Geometry check sheet. Reference: the model listing, model coordinates, mm. Face numbers are marked on the shaded views. A direction names the side the tool comes from. Round coordinates to 2 decimals unless told otherwise and drop trailing zeros. Write each loop counter-clockwise with the first axis right and the second up, starting at its lowest first coordinate (ties: lowest second). Pieces come first, ordered by that corner, then holes. Notation, with made-up numbers: M 79,64 L 135,64 A22 cw 135,87 Z; hole C 68,43.5 d8. An arc over 180 degrees is marked long. Put each result on its own line as item: value. Start each with the question number.
(1) Section check A-A on z = 64. Record the cut outline in (x, y).
(2) Mould release check, pull along Y, two halves, no side actions. Record for the marked faces 3, 4 and 5: pulls with the +Y half, pulls with the -Y half, needs draft (parallel to the pull), parting line crosses it, or undercut.
(3) Section check C-C on x = 37.5. Record the cut outline in (y, z).
(4) Gauge pin test, flat ends, axial feed: pin 1 (5 mm diameter, centred on x = 45, z = 17, fed in from -Y); pin 2 (4 mm diameter, centred on x = 4, z = 22.5, fed in from +Y); pin 3 (4 mm diameter, centred on x = 4, z = 27, fed in from -Y); pin 4 (3 mm diameter, centred on y = 33.5, z = 80.5, fed in from +X). Record the tip position at first contact, or that the pin passes through.
(5) Tool access check on the marked faces 1 and 2. Record the directions out of +Z, -Z, +X, -X, +Y, -Y that give a thin tool (end or side, any length) a straight path to the whole face; none if there is none.
(6) Section check D-D on z = 7. Record the cut outline in (x, y), then the cut area to 3 significant figures.
(7) Section check B-B on y = 36. Record the cut outline in (x, z).
(8) Material ranges on probe 1 along X at (y, z) = (4, 72.5); probe 2 along Z at (x, y) = (14.5, 33.5); probe 3 along X at (y, z) = (51, 35), recorded low to high.
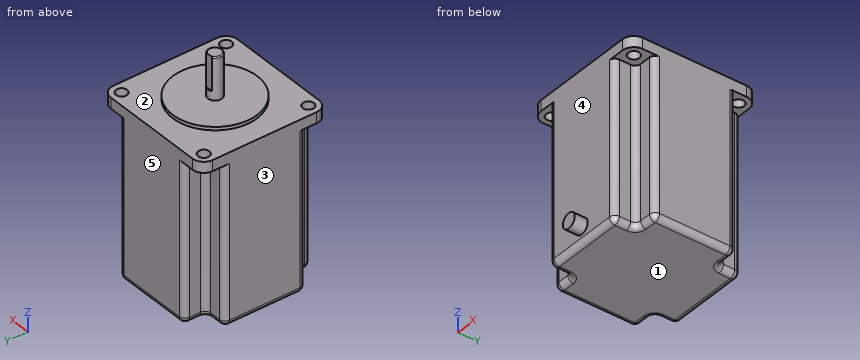
from build123d import *

# Parameters (mm, degrees)
SKETCH1_W           = 57.15
SKETCH1_H           = 57.15
BOSS_EXTRUDE1_DEPTH = 76.2
SKETCH2_R           = 19.05
BOSS_EXTRUDE2_DEPTH = 1.524
SKETCH3_R           = 3.175
BOSS_EXTRUDE3_DEPTH = 19.05
SKETCH18_W          = 20.32
SKETCH18_H          = 20.32
CUT_EXTRUDE13_DEPTH = 71.3232
SKETCH20_W          = 20.32
SKETCH20_H          = 20.32
CUT_EXTRUDE14_DEPTH = 71.3232
SKETCH21_W          = 20.32
SKETCH21_H          = 20.32
CUT_EXTRUDE15_DEPTH = 71.3232
SKETCH22_W          = 20.32
SKETCH22_H          = 20.32
CUT_EXTRUDE16_DEPTH = 71.3232
SKETCH11_R          = 2.54
CUT_EXTRUDE8_DEPTH  = 112.079633597
SKETCH12_R          = 2.54
CUT_EXTRUDE9_DEPTH  = 112.079633597
SKETCH14_R          = 2.54
CUT_EXTRUDE10_DEPTH = 112.079633597
SKETCH15_R          = 2.54
CUT_EXTRUDE11_DEPTH = 112.079633597
FILLET2_R           = 5.08
FILLET4_R           = 2.54
FILLET1_R           = 0.508
SKETCH10_W          = 7.148953117
SKETCH10_H          = 1.106198654
CUT_EXTRUDE7_DEPTH  = 14.986
SKETCH23_R          = 3.429
WIRE_2_DEPTH        = 5.842


with BuildPart() as part:
    # Sketch1 → Boss-Extrude1 (new body)
    with BuildSketch(Plane.XY):
        with Locations((28.575, 28.575)):
            Rectangle(SKETCH1_W, SKETCH1_H)
    extrude(amount=BOSS_EXTRUDE1_DEPTH)

    # Sketch2 → Boss-Extrude2 (add)
    with BuildSketch(Plane.XY.offset(76.2)):
        with Locations(Location((28.575, 28.575, 0), (0, 0, 180))):
            Circle(SKETCH2_R)
    extrude(amount=BOSS_EXTRUDE2_DEPTH)

    # Sketch3 → Boss-Extrude3 (add)
    with BuildSketch(Plane.XY.offset(77.724)):
        with Locations(Location((28.575, 28.575, 0), (0, 0, 180))):
            Circle(SKETCH3_R)
    extrude(amount=BOSS_EXTRUDE3_DEPTH)

    # Sketch18 → Cut-Extrude13 (cut)
    with BuildSketch(Plane(origin=(0, 0, 0), x_dir=(-1, 0, 0), z_dir=(0, 0, -1))):
        with Locations((0, 57.15)):
            Rectangle(SKETCH18_W, SKETCH18_H)
    extrude(amount=-CUT_EXTRUDE13_DEPTH, mode=Mode.SUBTRACT)

    # Sketch20 → Cut-Extrude14 (cut)
    with BuildSketch(Plane(origin=(0, 0, 0), x_dir=(-1, 0, 0), z_dir=(0, 0, -1))):
        Rectangle(SKETCH20_W, SKETCH20_H)
    extrude(amount=-CUT_EXTRUDE14_DEPTH, mode=Mode.SUBTRACT)

    # Sketch21 → Cut-Extrude15 (cut)
    with BuildSketch(Plane(origin=(0, 0, 0), x_dir=(-1, 0, 0), z_dir=(0, 0, -1))):
        with Locations((-57.15, 0)):
            Rectangle(SKETCH21_W, SKETCH21_H)
    extrude(amount=-CUT_EXTRUDE15_DEPTH, mode=Mode.SUBTRACT)

    # Sketch22 → Cut-Extrude16 (cut)
    with BuildSketch(Plane(origin=(0, 0, 0), x_dir=(-1, 0, 0), z_dir=(0, 0, -1))):
        with Locations((-57.15, 57.15)):
            Rectangle(SKETCH22_W, SKETCH22_H)
    extrude(amount=-CUT_EXTRUDE16_DEPTH, mode=Mode.SUBTRACT)

    # Sketch11 → Cut-Extrude8 (cut, through all)
    with BuildSketch(Plane.XY.offset(76.2)):
        with Locations((4.953, 52.233071325)):
            Circle(SKETCH11_R)
    extrude(amount=-CUT_EXTRUDE8_DEPTH, mode=Mode.SUBTRACT)

    # Sketch12 → Cut-Extrude9 (cut, through all)
    with BuildSketch(Plane.XY.offset(76.2)):
        with Locations((52.197, 52.233071325)):
            Circle(SKETCH12_R)
    extrude(amount=-CUT_EXTRUDE9_DEPTH, mode=Mode.SUBTRACT)

    # Sketch14 → Cut-Extrude10 (cut, through all)
    with BuildSketch(Plane.XY.offset(76.2)):
        with Locations((4.953, 4.989071325)):
            Circle(SKETCH14_R)
    extrude(amount=-CUT_EXTRUDE10_DEPTH, mode=Mode.SUBTRACT)

    # Sketch15 → Cut-Extrude11 (cut, through all)
    with BuildSketch(Plane.XY.offset(76.2)):
        with Locations((52.197, 4.989071325)):
            Circle(SKETCH15_R)
    extrude(amount=-CUT_EXTRUDE11_DEPTH, mode=Mode.SUBTRACT)

    # Fillet2
    fillet2_edges = [part.edges().sort_by_distance(p)[0] for p in [
        (0, 57.15, 73.7616),
        (57.15, 57.15, 73.7616),
        (57.15, 0, 73.7616),
        (0, 0, 73.7616),
    ]]
    fillet(fillet2_edges, radius=FILLET2_R)

    # Fillet4
    fillet4_edges = [part.edges().sort_by_distance(p)[0] for p in [
        (0, 28.575, 0),
        (10.16, 52.07, 0),
        (5.08, 46.99, 0),
        (0, 46.99, 35.6616),
        (10.16, 57.15, 35.6616),
        (10.16, 46.99, 35.6616),
        (28.575, 0, 0),
        (5.08, 10.16, 0),
        (10.16, 5.08, 0),
        (10.16, 0, 35.6616),
        (0, 10.16, 35.6616),
        (10.16, 10.16, 35.6616),
        (57.15, 28.575, 0),
        (46.99, 5.08, 0),
        (52.07, 10.16, 0),
        (57.15, 10.16, 35.6616),
        (46.99, 0, 35.6616),
        (46.99, 10.16, 35.6616),
        (28.575, 57.15, 0),
        (52.07, 46.99, 0),
        (46.99, 52.07, 0),
        (46.99, 57.15, 35.6616),
        (57.15, 46.99, 35.6616),
        (46.99, 46.99, 35.6616),
    ]]
    fillet(fillet4_edges, radius=FILLET4_R)

    # Fillet1
    fillet1_edges = [part.edges().sort_by_distance(p)[0] for p in [
        (31.75, 28.575, 96.774),
    ]]
    fillet(fillet1_edges, radius=FILLET1_R)

    # Sketch10 → Cut-Extrude7 (cut)
    with BuildSketch(Plane.XY.offset(96.774)):
        with Locations((29.031069878, 31.795099327)):
            Rectangle(SKETCH10_W, SKETCH10_H)
    extrude(amount=-CUT_EXTRUDE7_DEPTH, mode=Mode.SUBTRACT)

    # Sketch23 → Wire 2 (add)
    with BuildSketch(Plane.XZ):
        with Locations(Location((28.575, 7.343801428, 0), (0, 0, 90))):
            Circle(SKETCH23_R)
    extrude(amount=WIRE_2_DEPTH)


solid = part.part
Answers follow:
1. outline: M 0,12.7 A2.54 ccw 2.54,10.16 L 7.62,10.16 A2.54 cw 10.16,7.62 L 10.16,2.54 A2.54 ccw 12.7,0 L 44.45,0 A2.54 ccw 46.99,2.54 L 46.99,7.62 A2.54 cw 49.53,10.16 L 54.61,10.16 A2.54 ccw 57.15,12.7 L 57.15,44.45 A2.54 ccw 54.61,46.99 L 49.53,46.99 A2.54 cw 46.99,49.53 L 46.99,54.61 A2.54 ccw 44.45,57.15 L 12.7,57.15 A2.54 ccw 10.16,54.61 L 10.16,49.53 A2.54 cw 7.62,46.99 L 2.54,46.99 A2.54 ccw 0,44.45 Z
2. face 3: needs draft
2. face 4: pulls with the -Y half
2. face 5: pulls with the +Y half
3. outline: M 0,2.54 A2.54 ccw 2.54,0 L 54.61,0 A2.54 ccw 57.15,2.54 L 57.15,76.2 L 45.4,76.2 L 45.4,77.72 L 11.75,77.72 L 11.75,76.2 L 0,76.2 Z
4. pin 1: stops at y = 0
4. pin 2: stops at y = 46.99
4. pin 3: stops at y = 10.16
4. pin 4: passes through
5. face 1: -Z, +X, -X, +Y, -Y
5. face 2: +Z
6. outline: M 0,12.7 A2.54 ccw 2.54,10.16 L 7.62,10.16 A2.54 cw 10.16,7.62 L 10.16,2.54 A2.54 ccw 12.7,0 L 25.16,0 L 25.16,-5.84 L 31.99,-5.84 L 31.99,0 L 44.45,0 A2.54 ccw 46.99,2.54 L 46.99,7.62 A2.54 cw 49.53,10.16 L 54.61,10.16 A2.54 ccw 57.15,12.7 L 57.15,44.45 A2.54 ccw 54.61,46.99 L 49.53,46.99 A2.54 cw 46.99,49.53 L 46.99,54.61 A2.54 ccw 44.45,57.15 L 12.7,57.15 A2.54 ccw 10.16,54.61 L 10.16,49.53 A2.54 cw 7.62,46.99 L 2.54,46.99 A2.54 ccw 0,44.45 Z
6. area: 2,890 mm^2
7. outline: M 0,2.54 A2.54 ccw 2.54,0 L 54.61,0 A2.54 ccw 57.15,2.54 L 57.15,76.2 L 46.12,76.2 L 46.12,77.72 L 11.03,77.72 L 11.03,76.2 L 0,76.2 Z
8. probe 1: x = 0.12 to 2.61, 7.29 to 49.86, 54.54 to 57.03
8. probe 2: z = 0 to 77.72
8. probe 3: x = 10.16 to 46.99
